Part model, mm, in its own coordinate system. A direction names the side the tool comes from. Coordinates: 2 decimals unless noted, no trailing zeros. Write each loop counter-clockwise with the first axis right and the second up, starting at its lowest first coordinate (ties: lowest second). Pieces come first, ordered by that corner, then holes. Notation, with made-up numbers: (-35.75, 55) - (4.25, 55) arc R19 ccw to (4.25, 69) - close; hole circle Ø10 at (25.5, 42.5). An arc over 180 degrees is marked (long way). Use a Markdown table: item, result.
```python
from build123d import *

# Parameters (mm, degrees)
F0_R     = 19.05
F1_DEPTH = 25.4
F3_D     = 11.43
F4_R     = 15.367
F5_DEPTH = 3.175
F7_R     = 7.9375
F8_DEPTH = 19.05


with BuildPart() as f1:
    # F0 (on Top) → F1 (new body)
    with BuildSketch(Plane.XY):
        Circle(F0_R)
    extrude(amount=F1_DEPTH)

    # F3 (through all)
    with Locations(Plane.XY.offset(25.4)):
        with Locations((0, 0)):
            Hole(F3_D / 2)

    # F4 (on face) → F5 (cut)
    with BuildSketch(Plane.XY.offset(25.4)):
        Circle(F4_R)
    extrude(amount=-F5_DEPTH, mode=Mode.SUBTRACT)

    # F7 (on offset) → F8 (cut)
    with BuildSketch(Plane.XZ.offset(19.05)):
        with Locations((0, 12.7)):
            Circle(F7_R)
    extrude(amount=-F8_DEPTH, mode=Mode.SUBTRACT)


solid = f1.part
```
Item 1: Band-saw the part on D-D, the plane x = -7. Give the cut face in (y, z) (3 decimals).
From the geometry:
| item | result |
|---|---|
| outline | (-17.717, 0) - (17.717, 0) - (17.717, 25.4) - (13.68, 25.4) - (13.68, 22.225) - (-13.68, 22.225) - (-13.68, 25.4) - (-17.717, 25.4) - (-17.717, 16.442) - (0, 16.442) - (0, 8.958) - (-17.717, 8.958) - close |
Item 2: Which spindle directions (+Z, -Z, +X, -X, +Y, -Y) get a long thin tool onto all of the face, cutting with end or side? Do faces 4 (the face through (-2.48, 18.888, 12.522)), 5 (the face through (14.657, 4.616, 23.835)), 6 (the face through (7, 0, 13)). Say none if no direction does.
From the geometry:
| item | result |
|---|---|
| face 4 | +Z, -Z |
| face 5 | +Z |
| face 6 | -Y |
Item 3: Band-saw the part on C-C, the plane z = 2.75. Give the cut face in (x, y) (3 decimals), then the cut area to 3 significant figures.
From the geometry:
| item | result |
|---|---|
| outline | circle Ø38.1 at (0, 0); hole circle Ø11.43 at (0, 0) |
| area | 1,040 mm^2 |
Item 4: Drop flat-ended pins along their axis: P1, Ø1.5, axis at x = -7, z = 6, coming from the +Y side; P2, Ø3, axis at y = -4.5, z = 4.5, coming from the +X side; P3, Ø5, axis at y = 11.5, z = 20, coming from the +X side. Give the stop position or say it passes through.
From the geometry:
| item | result |
|---|---|
| P1 | y = 18 |
| P2 | x = 18.81 |
| P3 | x = 16.79 |
Item 5: Band-saw the part on B-B, the plane y = -10. Give the cut face in (x, z) (1 decimal).
From the geometry:
| item | result |
|---|---|
| outline | (-16.2, 0) - (16.2, 0) - (16.2, 25.4) - (11.7, 25.4) - (11.7, 22.2) - (-11.7, 22.2) - (-11.7, 25.4) - (-16.2, 25.4) - close; hole circle Ø15.9 at (0, 12.7) |
Item 6: Two-plate mould, pull along Z, no slides. Class faces 1 (the face through (4, 5, 0)), 2 (the face through (-7, 0, 13)), 3 (the face through (-13, 9, 25.4)): pulls with the +Z half, pulls with the -Z half, needs draft (parallel to the pull), parting line crosses it, or undercut.
From the geometry:
| item | result |
|---|---|
| face 1 | pulls with the -Z half |
| face 2 | undercut |
| face 3 | pulls with the +Z half |
Item 7: Band-saw the part on A-A, the plane x = 0. Count the separate pieces of the cut face and the enclosed holes in it, then the cut area to 3 significant figures.
From the geometry:
| item | result |
|---|---|
| separate pieces | 3 |
| enclosed holes | 0 |
| area | 404 mm^2 |
Item 8: Drill centre lines: probe 1 along Y at (x, z) = (0, 23.4); probe 2 along Y at (x, z) = (0, 12.5) (3 decimals); probe 3 along Z at (x, y) = (11, 4) (3 decimals). Where is each one in solid material? Low to high.
From the geometry:
| item | result |
|---|---|
| probe 1 | -19.05 to -15.37, 15.37 to 19.05 |
| probe 2 | 5.715 to 19.05 |
| probe 3 | 0 to 22.225 |
